from build123d import *

# Parameters (mm, degrees)
SKETCH1_R           = 2.5
SKETCH1_R_2         = 3.375
BOSS_EXTRUDE1_DEPTH = 6.35


with BuildPart() as part:
    # Sketch1 → Boss-Extrude1 (new body)
    with BuildSketch(Plane(origin=(0, 6.35, 0), x_dir=(1, 0, 0), z_dir=(0, 1, 0))):
        Polygon((25.4, 63.5), (0, 63.5), (0, 0), (63.5, 0), (63.5, 25.4), align=None)
        with Locations(Location((13.4512, 41.304668328, 0), (0, 0, 90))):
            Circle(SKETCH1_R, mode=Mode.SUBTRACT)
        with Locations(Location((11.9488, 60.295331672, 0), (0, 0, 90))):
            Circle(SKETCH1_R, mode=Mode.SUBTRACT)
        with Locations(Location((11.9488, 22.195331672, 0), (0, 0, 90))):
            Circle(SKETCH1_R, mode=Mode.SUBTRACT)
        with Locations(Location((13.4512, 3.204668328, 0), (0, 0, 90))):
            Circle(SKETCH1_R, mode=Mode.SUBTRACT)
        with Locations(Location((22.195331672, 13.4512, 0), (0, 0, 90))):
            Circle(SKETCH1_R, mode=Mode.SUBTRACT)
        with Locations(Location((3.204668328, 11.9488, 0), (0, 0, 90))):
            Circle(SKETCH1_R, mode=Mode.SUBTRACT)
        with Locations(Location((41.304668328, 11.9488, 0), (0, 0, 90))):
            Circle(SKETCH1_R, mode=Mode.SUBTRACT)
        with Locations(Location((60.295331672, 13.4512, 0), (0, 0, 90))):
            Circle(SKETCH1_R, mode=Mode.SUBTRACT)
        with Locations(Location((12.7, 50.8, 0), (0, 0, 90))):
            Circle(SKETCH1_R_2, mode=Mode.SUBTRACT)
        with Locations(Location((12.7, 31.75, 0), (0, 0, 90))):
            Circle(SKETCH1_R_2, mode=Mode.SUBTRACT)
        with Locations(Location((50.8, 12.7, 0), (0, 0, 90))):
            Circle(SKETCH1_R_2, mode=Mode.SUBTRACT)
        with Locations(Location((31.75, 12.7, 0), (0, 0, 90))):
            Circle(SKETCH1_R_2, mode=Mode.SUBTRACT)
        with Locations(Location((12.7, 12.7, 0), (0, 0, 90))):
            Circle(SKETCH1_R_2, mode=Mode.SUBTRACT)
    extrude(amount=-BOSS_EXTRUDE1_DEPTH)


solid = part.part
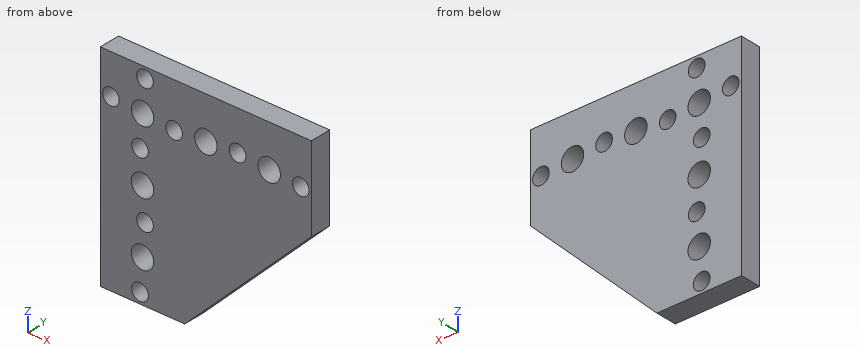
Input: part model. Units: mm. Frame: model coordinates. Coordinates: 2 decimals unless noted, no trailing zeros. Loops run counter-clockwise (first coordinate to the right, second up) from the corner with the lowest first, then second, coordinate; pieces in that order, holes last. Notation, with made-up numbers: (35.25, 10.5) - (82.25, 10.5) arc R18 ccw to (82.25, 16.5) - close; hole circle Ø11 at (83.5, 10). An arc over 180 degrees is marked (long way). Answer in a Markdown table with one row per item. Add a question column.
Item 1: Contact query for flat-ended pins moving along their axis: P1, Ø2, axis at y = 4, z = -56, coming from the +X side; P2, Ø4, axis at x = 41.3, z = -11.95, coming from the +Y side. Output: stop coordinate, or through.
Item 2: Section query A-A on x = 50.8. Return the cut outline in (y, z) (3 decimals), then the cut area to 3 significant figures.
Item 3: Section query C-C on z = -12.7. State how many separate pieces and enclosed holes the cut face has, then the cut area to 3 significant figures.
Item 4: Line query: line 1 along X through (y, z) = (1.5, -22.5); line 2 along Z through (x, y) = (21.5, 6); line 3 along Z through (x, y) = (61.5, 1). Output: solid intervals per line, ascending. Write a range as [from, to].
Item 5: Section query B-B on z = -31.75. Return the cut outline in (x, y) (3 decimals).
Recorded:
| question | item | result |
|---|---|---|
| 1 | P1 | x = 33.9 |
| 1 | P2 | through |
| 2 | outline | (0, -38.1) - (6.35, -38.1) - (6.35, -16.075) - (0, -16.075) - close; (0, -9.325) - (6.35, -9.325) - (6.35, 0) - (0, 0) - close |
| 2 | area | 199 mm^2 |
| 3 | separate pieces | 8 |
| 3 | enclosed holes | 0 |
| 3 | area | 154 mm^2 |
| 4 | line 1 | [0, 9.47], [14.43, 63.5] |
| 4 | line 2 | [-63.5, -15.85], [-11.05, 0] |
| 4 | line 3 | [-27.4, -15.64], [-11.26, 0] |
| 5 | outline | (0, 0) - (9.325, 0) - (9.325, 6.35) - (0, 6.35) - close; (16.075, 0) - (57.15, 0) - (57.15, 6.35) - (16.075, 6.35) - close |
